Part model, mm, in its own coordinate system. Round coordinates to 2 decimals unless told otherwise and drop trailing zeros. Order: outer loops, then holes, each group sorted by start corner. A loop starts at its lowest first (then second) coordinate and runs counter-clockwise, first axis right, second up. Notation, with made-up numbers: (17, 11) -> (59, 11) arc R32 cw to (59, 49) -> close; hole circle Ø1 at (-11, 27.5). An arc over 180 degrees is marked (long way). Use CSV: the item, a comma, the result in double quotes.
```python
from build123d import *

# Parameters (mm, degrees)
EXTRUDE_1_DEPTH = 6


with BuildPart() as part:
    # Эскиз1 → Бобышка-Вытянуть1 (new body)
    with BuildSketch(Plane.XY):
        with BuildLine():
            Line((82.05, 82.05), (0, 82.05))
            Line((0, 82.05), (0, 69.05))
            ThreePointArc((0, 69.05), (48.825723241, 48.825723241), (69.05, 0))
            ThreePointArc((69.05, 0), (48.825723241, -48.825723241), (0, -69.05))
            Line((0, -69.05), (0, -82.05))
            Line((0, -82.05), (82.05, -82.05))
            Line((82.05, -82.05), (82.05, 82.05))
        make_face()
    extrude(amount=EXTRUDE_1_DEPTH)


solid = part.part
```
(1) Cut at A-A, the plane x = 44. Give the cut face in (y, z), then the cut area to 3 significant figures.
Reply:
outline,"(-82.05, 0) -> (-53.22, 0) -> (-53.22, 6) -> (-82.05, 6) -> close; (53.22, 0) -> (82.05, 0) -> (82.05, 6) -> (53.22, 6) -> close"
area,"346 mm2"
(2) Drop flat-ended pins along their axis: P1, Ø2, axis at y = -56.5, z = 4, coming from the -X side; P2, Ø1, axis at y = -57.5, z = 1.5, coming from the -X side; P3, Ø8, axis at x = 72, y = -50, coming from the -Z side. Give the stop position or say it passes through.
Reply:
P1,"x = 38.23"
P2,"x = 37.47"
P3,"z = 0"
(3) Cut at B-B, the plane z = 2.05. Give the cut face in (x, y), then the cut area to 4 significant figures.
Reply:
outline,"(0, -82.05) -> (82.05, -82.05) -> (82.05, 82.05) -> (0, 82.05) -> (0, 69.05) arc R69.05 cw to (0, -69.05) -> close"
area,"5,975 mm2"
(4) Probe probe 1 along Y at (x, z) = (16.5, 1); probe 2 along Y at (x, z) = (40, 1.8); probe 3 along X at (y, z) = (59.5, 0.75). List the from-to ranges inside material, lowest first. Write a range as [from, to].
Reply:
probe 1,"[-82.05, -67.05], [67.05, 82.05]"
probe 2,"[-82.05, -56.28], [56.28, 82.05]"
probe 3,"[35.04, 82.05]"
(5) Cut at D-D, the plane y = -28. Give the cut face in (x, z).
Reply:
outline,"(63.12, 0) -> (82.05, 0) -> (82.05, 6) -> (63.12, 6) -> close"
(6) Cut at C-C, the plane x = 11.5. Give the cut face in (y, z), then the cut area to 3 significant figures.
Reply:
outline,"(-82.05, 0) -> (-68.09, 0) -> (-68.09, 6) -> (-82.05, 6) -> close; (68.09, 0) -> (82.05, 0) -> (82.05, 6) -> (68.09, 6) -> close"
area,"168 mm2"
